Source: CAD feature listing. Evaluate the final solid. Frame: model axes, mm. Face numbers are marked on the shaded views. A direction names the side the tool comes from. Round coordinates to 2 decimals unless told otherwise and drop trailing zeros. Order: outer loops, then holes, each group sorted by start corner. A loop starts at its lowest first (then second) coordinate and runs counter-clockwise, first axis right, second up. Notation, with made-up numbers: (-33, 73) -> (16, 73) arc R10 ccw to (16, 80) -> close; hole circle Ø11 at (-0.5, 0). An arc over 180 degrees is marked (long way). One line per item, written item: value. Start each with the question number.
1) Reachability of the marked faces 1, 2 and 3 from +Z, -Z, +X, -X, +Y, -Y: full face, straight path, thin tool, end or side. Return the list, or none.
2) Mould query, pull axis X, two halves, no side actions, for the marked faces 4, 5 and 6. Classes: pulls with the +X half, pulls with the -X half, needs draft (parallel to the pull), parting line crosses it, or undercut.
3) Section C-C (x = -148.5). Return the cut outline in (y, z).
4) Section B-B (y = 22). Return the cut outline in (x, z), and give its area (3 significant figures).
5) Ray query, L1, parallel to Z at x = -78.5, y = 26.5; L2, parallel to Y at x = -38, z = 24; L3, parallel to X at y = 12, z = 43. Return the intervals inside material, ascending.
6) Section A-A (z = -4). Return the cut outline in (x, y).
7) Pin query (flat end, axial travel): P1, Ø2.5, axis at y = 38, z = -7.5, coming from the -X side; P2, Ø8, axis at x = -84.5, y = 36, coming from the +Z side; P3, Ø2, axis at x = -20.5, y = 35, coming from the -Z side. Return the tip coordinate at first contact, or that it passes through.
8) Section D-D (x = -112.5). Return the cut outline in (y, z), and give its area (3 significant figures).
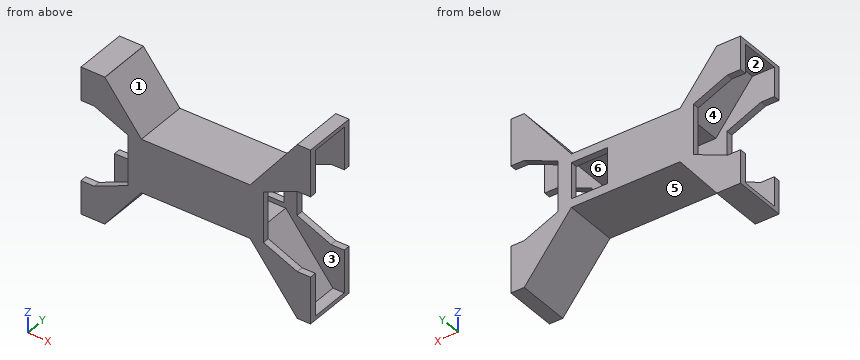
Autodesk Inventor part; units mm, degrees
ref_plane "YZ Plane" through (0, 0, 0) normal (1, 0, 0) x (0, 1, 0)
ref_plane "XZ Plane" through (0, 0, 0) normal (0, 1, 0) x (-1, 0, 0)
ref_plane "XY Plane" through (0, 0, 0) normal (0, 0, 1) x (1, 0, 0)
sketch "Sketch1" plane through (0, 0, 0) normal (0, 1, 0) x (-1, 0, 0)
  line L0 (172.412, 0) -> (172.412, -65)
  line L1 (172.412, 0) -> (172.412, 65)
  line L2 (172.412, 65) -> (162.412, 65)
  line L3 (162.412, 65) -> (127.012, 20)
  line L4 (172.412, -65) -> (162.412, -65)
  line L5 (162.412, -65) -> (127.012, -20)
  line L6 (127.012, -20) -> (86.206, -20)
  line L7 (127.012, 20) -> (86.206, 20)
  line L8 (0, 0) -> (0, -65)
  line L9 (0, 0) -> (0, 65)
  line L10 (0, 65) -> (10, 65)
  line L11 (10, 65) -> (45.4, 20)
  line L12 (0, -65) -> (10, -65)
  line L13 (10, -65) -> (45.4, -20)
  line L14 (45.4, -20) -> (86.206, -20)
  line L15 (45.4, 20) -> (86.206, 20)
  dimension "d0" = 172.412
  dimension "d1" = 65
  dimension "d2" = 65
  dimension "d7" = 10
extrude "Extrusion1" add sketch "Sketch1" along normal blind 5
sketch "Sketch2" plane through (0, 5, 0) normal (0, 1, 0) x (1, 0, 0)
  line L0 (-162.412, -65) -> (-127.012, -20)
  line L1 (-127.012, -20) -> (-162.412, -65)
  line L2 (-162.412, -65) -> (-172.412, -65)
  line L3 (-127.012, 20) -> (-162.412, 65)
  line L4 (-172.412, 65) -> (-162.412, 65)
  line L5 (-162.412, 65) -> (-127.012, 20)
  line L6 (-127.012, 20) -> (-45.4, 20)
  line L7 (-10, 65) -> (-45.4, 20)
  line L8 (-45.4, 20) -> (-10, 65)
  line L9 (-10, 65) -> (0, 65)
  line L10 (0, -65) -> (0, 65)
  line L11 (-45.4, -20) -> (-10, -65)
  line L12 (0, -65) -> (-10, -65)
  line L13 (-10, -65) -> (-45.4, -20)
  line L14 (-45.4, -20) -> (-127.012, -20)
  line L15 (-128.469, -17) -> (-163.869, -62)
  line L16 (-163.869, -62) -> (-169.412, -62)
  line L17 (-169.412, 62) -> (-163.869, 62)
  line L18 (-163.869, 62) -> (-128.469, 17)
  line L19 (-128.469, 17) -> (-43.943, 17)
  line L20 (-43.943, 17) -> (-8.543, 62)
  line L21 (-8.543, 62) -> (-3, 62)
  line L22 (-3, -62) -> (-8.543, -62)
  line L23 (-8.543, -62) -> (-43.943, -17)
  line L24 (-43.943, -17) -> (-128.469, -17)
  line L25 (-3, -62) -> (0, -62)
  line L26 (0, -65) -> (0, -62)
  line L27 (-3, 62) -> (0, 62)
  line L28 (0, 65) -> (0, 62)
  line L29 (-169.412, -62) -> (-172.412, -62)
  line L30 (-172.412, -65) -> (-172.412, -62)
  line L31 (-169.412, 62) -> (-172.412, 62)
  line L32 (-172.412, 62) -> (-172.412, 65)
  point P0 (0, 0)
  dimension "d10" = 3
extrude "Extrusion2" add sketch "Sketch2" along normal blind 30
sketch "Sketch3" plane through (0, 35, 0) normal (0, 1, 0) x (1, 0, 0)
  line L0 (-172.412, 65) -> (-172.412, -65)
  line L1 (-172.412, -65) -> (-172.412, 65)
  line L2 (-162.412, 65) -> (-172.412, 65)
  line L3 (-172.412, 65) -> (-162.412, 65)
  line L4 (-45.4, 20) -> (-127.012, 20)
  line L5 (-162.412, 65) -> (-127.012, 20)
  line L6 (-127.012, 20) -> (-45.4, 20)
  line L7 (-45.4, 20) -> (-10, 65)
  line L8 (0, 65) -> (-10, 65)
  line L9 (-10, 65) -> (0, 65)
  line L10 (-10, -65) -> (0, -65)
  line L11 (0, 65) -> (0, -65)
  line L12 (0, -65) -> (-10, -65)
  line L13 (-127.012, -20) -> (-45.4, -20)
  line L14 (-10, -65) -> (-45.4, -20)
  line L15 (-45.4, -20) -> (-127.012, -20)
  line L16 (-162.412, -65) -> (-127.012, -20)
  line L17 (-127.012, -20) -> (-162.412, -65)
  line L18 (-172.412, -65) -> (-162.412, -65)
  line L19 (-162.412, -65) -> (-172.412, -65)
  point P0 (0, 0)
extrude "Extrusion3" add sketch "Sketch3" along normal blind 5
sketch "Sketch4" plane through (0, 40, 0) normal (0, 1, 0) x (1, 0, 0)
  line L0 (0, 0) -> (0, -30)
  line L1 (0, -62) -> (0, 62)
  line L2 (0, 0) -> (0, 30)
  line L3 (0, 30) -> (-10, 30)
  line L4 (-35.4, 0) -> (-35.4, 18.85)
  line L5 (-35.4, 18.85) -> (-10, 30)
  line L6 (-35.4, 0) -> (-35.4, -18.85)
  line L7 (-35.4, -18.85) -> (-10, -30)
  line L8 (-10, -30) -> (0, -30)
  line L9 (-127.012, -20) -> (-45.4, -20)
  line L10 (-45.4, 20) -> (-127.012, 20)
  line L11 (-172.412, 0) -> (-172.412, -30)
  line L12 (-172.412, 0) -> (-172.412, 30)
  line L13 (-172.412, 30) -> (-162.412, 30)
  line L14 (-137.012, 0) -> (-137.012, 18.85)
  line L15 (-137.012, 18.85) -> (-162.412, 30)
  line L16 (-137.012, 0) -> (-137.012, -18.85)
  line L17 (-137.012, -18.85) -> (-162.412, -30)
  line L18 (-162.412, -30) -> (-172.412, -30)
  dimension "d15" = 30
  dimension "d16" = 30
  dimension "d17" = 10
  dimension "d18" = 35.4
  dimension "d19" = 18.85
  dimension "d20" = 18.85
extrude "Extrusion4" cut sketch "Sketch4" against normal through all
sketch "Sketch5" plane through (0, 40, 0) normal (0, 1, 0) x (1, 0, 0)
  line L0 (-172.412, -65) -> (-162.412, -65)
  line L1 (-172.412, -65) -> (-172.412, -55)
  line L2 (-172.412, -30) -> (-172.412, -65)
  line L3 (-162.412, 65) -> (-172.412, 65)
  line L4 (-172.412, 65) -> (-172.412, 55)
  line L5 (-172.412, 65) -> (-172.412, 30)
  line L6 (-172.412, 55) -> (-154.5453, 55)
  line L7 (-127.012, 20) -> (-162.412, 65)
  line L8 (-172.412, -55) -> (-154.5453, -55)
  line L9 (-162.412, -65) -> (-127.012, -20)
  point P0 (0, 0)
  dimension "d23" = 10
  dimension "d24" = 10
extrude "Extrusion5" cut sketch "Sketch5" against normal through all
sketch "Sketch6" plane through (-172.412, 35, 30) normal (-1, 0, 0) x (0, 0, 1)
  line L0 (-85, 5) -> (-60, 5)
  line L1 (-50, -35) -> (-85, -35)
  line L2 (-85, 5) -> (-82, 5)
  line L3 (-82, 5) -> (-82, -35)
  line L4 (-82, -35) -> (-85, -35)
  line L5 (-85, -35) -> (-85, 5)
  line L6 (25, -35) -> (-10, -35)
  line L7 (25, 5) -> (22, 5)
  line L8 (22, 5) -> (22, -35)
  line L9 (22, -35) -> (25, -35)
  line L10 (25, -35) -> (25, 5)
  point P0 (-30, -35)
  dimension "d27" = 3
  dimension "d28" = 3
extrude "Extrusion6" add sketch "Sketch6" against normal blind 18
sketch "Sketch7" plane through (0, 40, 0) normal (0, 1, 0) x (1, 0, 0)
  line L0 (-35.4, 18.85) -> (-35.4, -18.85)
  line L1 (-45.4, 13.5) -> (-72.4, 13.5)
  line L2 (-72.4, 13.5) -> (-72.4, -13.5)
  line L3 (-72.4, -13.5) -> (-45.4, -13.5)
  line L4 (-45.4, -13.5) -> (-45.4, 13.5)
  point P0 (0, 0)
  dimension "d33" = 27
  dimension "d34" = 27
extrude "Extrusion7" cut sketch "Sketch7" against normal blind 18
properties part number "Metal_Shroud"
Findings:
1. face 1: +Z, +Y, -Y
1. face 2: -X
1. face 3: none
2. face 4: pulls with the -X half
2. face 5: undercut
2. face 6: needs draft
3. outline: (0, -47.32) -> (40, -47.32) -> (40, -23.89) -> (35, -23.89) -> (35, -42.46) -> (5, -42.46) -> (5, -23.89) -> (0, -23.89) -> close; (0, 23.89) -> (5, 23.89) -> (5, 42.46) -> (35, 42.46) -> (35, 23.89) -> (40, 23.89) -> (40, 47.32) -> (0, 47.32) -> close
4. outline: (-172.41, -55) -> (-154.41, -55) -> (-154.41, -54.83) -> (-127.01, -20) -> (-45.4, -20) -> (-10, -65) -> (0, -65) -> (0, -62) -> (-8.54, -62) -> (-43.94, -17) -> (-128.47, -17) -> (-156, -52) -> (-172.41, -52) -> close; (-172.41, 52) -> (-156, 52) -> (-128.47, 17) -> (-43.94, 17) -> (-8.54, 62) -> (0, 62) -> (0, 65) -> (-10, 65) -> (-45.4, 20) -> (-127.01, 20) -> (-154.41, 54.83) -> (-154.41, 55) -> (-172.41, 55) -> close
4. area: 1,270 mm2
5. L1: -20 to -17, 17 to 20
5. L2: 0 to 5, 35 to 40
5. L3: -148.92 to -145.11, -27.31 to -23.49
6. outline: (-137.01, 0) -> (-35.4, 0) -> (-35.4, 5) -> (-137.01, 5) -> close; (-137.01, 35) -> (-72.4, 35) -> (-72.4, 40) -> (-137.01, 40) -> close; (-45.4, 35) -> (-35.4, 35) -> (-35.4, 40) -> (-45.4, 40) -> close
7. P1: x = -137.01
7. P2: z = 20
7. P3: z = -52.92
8. outline: (0, -20) -> (40, -20) -> (40, 20) -> (0, 20) -> close; hole (5, -17) -> (35, -17) -> (35, 17) -> (5, 17) -> close
8. area: 580 mm2
